Autodesk Inventor part; units mm, degrees
ref_plane "YZ Plane" through (0, 0, 0) normal (1, 0, 0) x (0, 1, 0)
ref_plane "XZ Plane" through (0, 0, 0) normal (0, 1, 0) x (-1, 0, 0)
ref_plane "XY Plane" through (0, 0, 0) normal (0, 0, 1) x (1, 0, 0)
sketch "Sketch1" plane through (0, 0, 0) normal (1, 0, 0) x (0, 1, 0)
  line L0 (0, 0) -> (22.225, 0)
  line L1 (25.4, -3.175) -> (25.4, -25.4)
  line L2 (22.2268, -25.4) -> (22.2268, -6.3482)
  line L3 (19.0518, -3.1732) -> (0, -3.1732)
  line L4 (25.4, -25.4) -> (22.2268, -25.4)
  line L5 (0, 0) -> (0, -3.1732)
  arc A0 (25.4, -3.175) -> (22.225, 0) centre (22.225, -3.175) ccw
  arc A1 (22.2268, -6.3482) -> (19.0518, -3.1732) centre (19.0518, -6.3482) ccw
  point P0 (25.4, 0)
  dimension "d0" = 25.4
  dimension "d1" = 25.4
  dimension "d2" = 3.175
extrude "Extrusion1" add sketch "Sketch1" along normal blind 609.6
sketch "Sketch2" plane through (0, 0, 0) normal (0, 0, 1) x (1, 0, 0)
  line L0 (0, 0) -> (0, 22.225)
  circle A0 centre (12.7, 11.1125) radius 1.9225
  dimension "d5" = 12.7
hole "Hole1" at (12.7, 11.1125, 0) direction (0, 0, -1) diameter 6.35 end through all
pattern_linear "Rectangular Pattern1" count 24 spacing 25.4 along (1, 0, 0) of "Hole1"
sketch "Sketch3" plane through (0, 25.4, -3.175) normal (0, 1, 0) x (1, 0, 0)
  line L0 (0, 0) -> (0, 22.225)
  circle A0 centre (12.7, 11.1125) radius 5.2364
  point P0 (0, -3.175)
  dimension "d16" = 12.7
hole "Hole2" at (12.7, 25.4, -14.2875) direction (0, -1, 0) diameter 6.35 end through all
pattern_linear "Rectangular Pattern2" count 24 spacing 25.4 along (1, 0, 0) of "Hole2"
properties part number "frame_angle_horiz" material "Steel, Mild"
Part model, mm, in its own coordinate system. A direction names the side the tool comes from. Coordinates: 2 decimals unless noted, no trailing zeros. Write each loop counter-clockwise with the first axis right and the second up, starting at its lowest first coordinate (ties: lowest second). Pieces come first, ordered by that corner, then holes. Notation, with made-up numbers: (64, -7.75) - (79, -7.75) arc R13 ccw to (79, 4.25) - close; hole circle Ø2 at (12, 31.5). An arc over 180 degrees is marked (long way). Put each result on its own line as item: value.
1. Band-saw the part on A-A (x = 124.5). Write the cut outline in (y, z) (3 decimals).
Final values:
outline: (0, -3.173) - (19.052, -3.173) arc R3.175 cw to (22.227, -6.348) - (22.227, -25.4) - (25.4, -25.4) - (25.4, -3.175) arc R3.175 ccw to (22.225, 0) - (0, 0) - close
2. Flat gauge pins, fed straight in: pin 1 Ø8.5 at (x, z) = (342.9, -14.29) entering from -Y; pin 2 Ø8.5 at (x, y) = (495.3, 11.11) entering from -Z; pin 3 Ø8.5 at (x, z) = (190.5, -14.29) entering from +Y; pin 4 Ø3 at (x, z) = (383, -6) entering from -Y. Where does each tip first touch, or does it go through?
Final values:
pin 1: stops at y = 22.23
pin 2: stops at z = -3.17
pin 3: stops at y = 25.4
pin 4: stops at y = 21.63
3. 3-axis set-ups, long thin cutter, end or side, ignore diameter. For faces 1 (the flat face through (301, 10, -3.173)), 2 (the flat face through (0, 18, -2)): which of +Z, -Z, +X, -X, +Y, -Y reach the whole face in a straight line?
Final values:
face 1: -Z, +X, -X, -Y
face 2: +Z, -Z, -X, +Y, -Y
4. Probe line 1 along Y through (x, z) = (489.5, -20.25); line 2 along Z through (x, y) = (215.9, 23.5); line 3 along Y through (x, z) = (520.7, -1.25). List the from-to ranges inside material, lowest first. Write a range as [from, to].
Final values:
line 1: y = [22.23, 25.4]
line 2: z = [-25.4, -17.46], [-11.11, -0.27]
line 3: y = [0, 7.94], [14.29, 24.75]
